Build history of the part. All positions in model axes, mm. Round coordinates to 2 decimals unless told otherwise and drop trailing zeros. Write each loop counter-clockwise with the first axis right and the second up, starting at its lowest first coordinate (ties: lowest second). Pieces come first, ordered by that corner, then holes. Notation, with made-up numbers: (11, 52) - (64, 52) arc R17 cw to (64, 69) - close; hole circle Ø2 at (-27.5, 73). An arc over 180 degrees is marked (long way). One line per question, with ' | ' between items.
from build123d import *

# Parameters (mm, degrees)
BOSS_EXTRUDE1_DEPTH = 5
SKETCH2_W           = 149
SKETCH2_H           = 21.5
CUT_EXTRUDE1_DEPTH  = 6
SKETCH3_W           = 145.97
SKETCH3_H           = 1.85
CUT_EXTRUDE2_DEPTH  = 6
CUT_EXTRUDE4_DEPTH  = 6
LPATTERN1_COUNT     = 46
LPATTERN1_PITCH     = 3.2
SKETCH5_R           = 1.95
CUT_EXTRUDE5_DEPTH  = 10


with BuildPart() as part:
    # Sketch1 → Boss-Extrude1 (new body)
    with BuildSketch(Plane.XY):
        with BuildLine():
            Line((2, 0), (163, 0))
            ThreePointArc((163, 0), (164.414213562, -0.585786438), (165, -2))
            Line((165, -2), (165, -31.22))
            ThreePointArc((165, -31.22), (164.414213562, -32.634213562), (163, -33.22))
            Line((163, -33.22), (2, -33.22))
            ThreePointArc((2, -33.22), (0.585786438, -32.634213562), (0, -31.22))
            Line((0, -31.22), (0, -2))
            ThreePointArc((0, -2), (0.585786438, -0.585786438), (2, 0))
        make_face()
    extrude(amount=BOSS_EXTRUDE1_DEPTH)

    # Sketch2 → Cut-Extrude1 (cut, through all)
    with BuildSketch(Plane.XY.offset(5)):
        with Locations((82.5, -18.75)):
            Rectangle(SKETCH2_W, SKETCH2_H)
    extrude(amount=-CUT_EXTRUDE1_DEPTH, mode=Mode.SUBTRACT)

    # Sketch3 → Cut-Extrude2 (cut, through all)
    with BuildSketch(Plane.XY.offset(5)):
        with Locations((82.335, -7.075)):
            Rectangle(SKETCH3_W, SKETCH3_H)
    extrude(amount=-CUT_EXTRUDE2_DEPTH, mode=Mode.SUBTRACT)

    # Sketch4 → Cut-Extrude4 (cut, through all)
    with BuildSketch(Plane.XY.offset(5)):
        Polygon((155.735, -3.249176841), (156.5, -6.15), (154.14, -6.15), (154.905, -3.249176841), align=None)
    cut_extrude4 = extrude(amount=-CUT_EXTRUDE4_DEPTH, mode=Mode.SUBTRACT)

    # LPattern1: Cut-Extrude4 ×46
    with Locations(*[(-i * LPATTERN1_PITCH, 0, 0) for i in range(1, LPATTERN1_COUNT)]):
        add(cut_extrude4, mode=Mode.SUBTRACT)

    # Sketch5 → Cut-Extrude5 (cut)
    with BuildSketch(Plane.XY.offset(5)):
        with Locations((4, -11.61)):
            Circle(SKETCH5_R)
        with Locations((4, -21.61)):
            Circle(SKETCH5_R)
        with Locations((161, -11.61)):
            Circle(SKETCH5_R)
        with Locations((161, -21.61)):
            Circle(SKETCH5_R)
    extrude(amount=-CUT_EXTRUDE5_DEPTH, mode=Mode.SUBTRACT)


solid = part.part
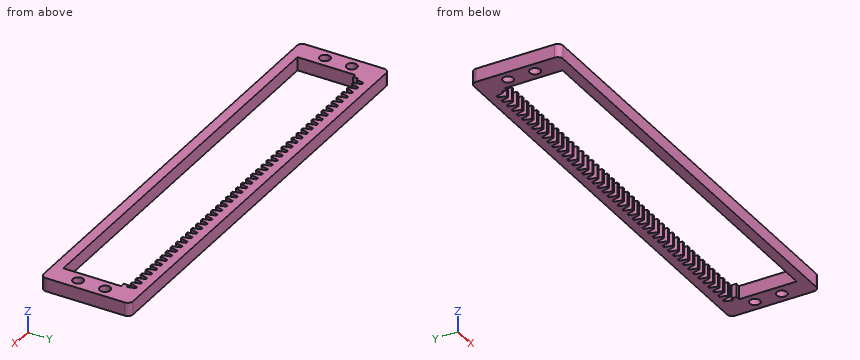
Q1. Saw through at A-A, the plane y = -11.61. List the corners of the cut face in (x, z).
Found:
outline: (0, 0) - (2.05, 0) - (2.05, 5) - (0, 5) - close; (5.95, 0) - (8, 0) - (8, 5) - (5.95, 5) - close; (157, 0) - (159.05, 0) - (159.05, 5) - (157, 5) - close; (162.95, 0) - (165, 0) - (165, 5) - (162.95, 5) - close
Q2. Drill centre lines: L1, parallel to X at y = -11.5, z = 4.6; L2, parallel to Y at x = 4, z = 2.8; L3, parallel to X at y = -9, z = 4.4. Where is each one in solid material? Low to high. Write a range as from..to.
Found:
L1: 0..2.05, 5.95..8, 157..159.05, 162.95..165 | L2: -33.22..-23.56, -19.66..-13.56, -9.66..0 | L3: 0..8, 157..165
Q3. Drop a flat-ended pin along its axis: pin 1 (5 mm diameter, centred on x = 91, y = -10, fed in from -Z). Give the stop position or say it passes through.
Found:
pin 1: through
Q4. Saw through at C-C, the plane z = 2.3. State how many separate pieces and enclosed holes the cut face has, then the cut area to 3 significant figures.
Found:
separate pieces: 1 | enclosed holes: 5 | area: 1,740 mm^2
Q5. Saw through at B-B, the plane x = 4. List the corners of the cut face in (y, z), then the cut area to 3 significant figures.
Found:
outline: (-33.22, 0) - (-23.56, 0) - (-23.56, 5) - (-33.22, 5) - close; (-19.66, 0) - (-13.56, 0) - (-13.56, 5) - (-19.66, 5) - close; (-9.66, 0) - (0, 0) - (0, 5) - (-9.66, 5) - close | area: 127 mm^2
